Print and shaded views of the part. All mm, measured from the part's lowest x, y and z. Give positions to 0.01 mm unless a question says otherwise; leave off trailing zeros. Write each loop counter-clockwise with the first axis right and the second up, starting at its lowest first coordinate (ties: lowest second). Pieces come first, ordered by that corner, then holes. Notation, with made-up numbers: M 9,21 L 32,21 A29 cw 32,57 Z; hole C 46,15 d1. An arc over 180 degrees is marked long. One line per question, with ' | ' between items. Start each with the question number.
1. Wall check: L1, parallel to Y at x = 31, z = 1.4; L2, parallel to X at y = 12, z = 3.1; L3, parallel to X at y = 14, z = 1.95. Give the ranges that are in metal, low to high.
2. Flat gauge pins, fed straight in: pin 1 (3.5 mm diameter, centred on x = 39.5, y = 17.5, fed in from +Z); pin 2 (8 mm diameter, centred on x = 12.5, y = 25, fed in from +Z). Where does each tip first touch, or does it go through?
3. Cut at D-D, the plane y = 8. Write the cut outline in (x, z).
4. Cut at A-A, the plane z = 0.45. Write the cut outline in (x, y).
5. Cut at C-C, the plane x = 23.5. Write the cut outline in (y, z), then the cut area to 3 significant figures.
6. Cut at B-B, the plane y = 17.5. Write the cut outline in (x, z).
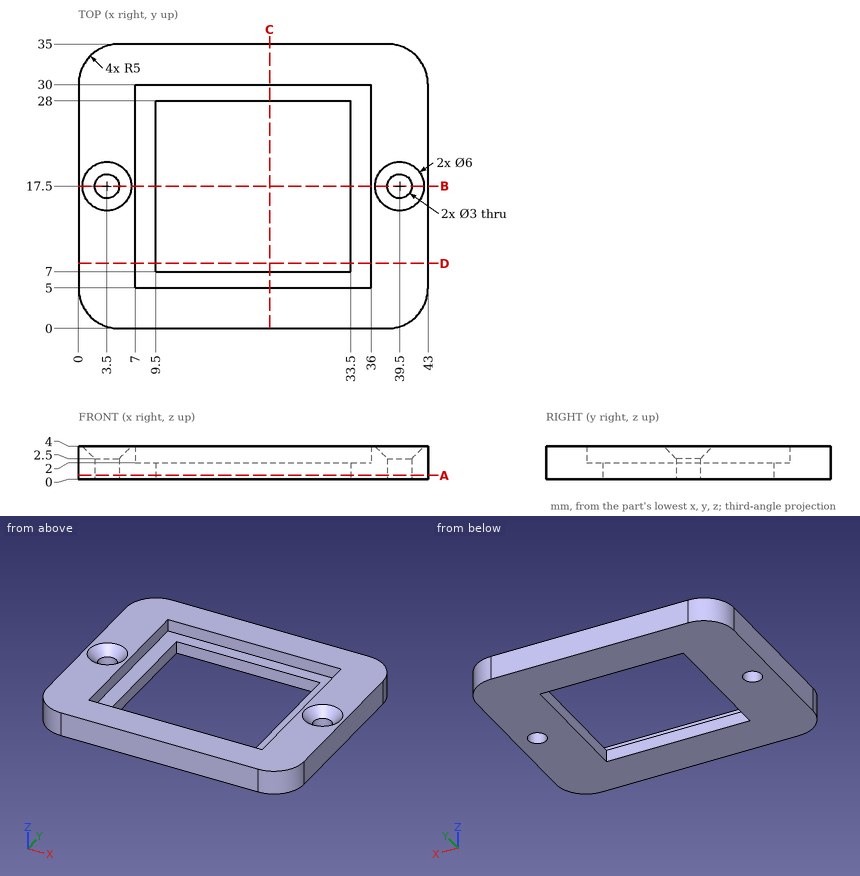
Here are the results:
1) L1: 0 to 7, 28 to 35 | L2: 0 to 7, 36 to 43 | L3: 0 to 9.5, 33.5 to 43
2) pin 1: z = 2.75 | pin 2: z = 2
3) outline: M 0,0 L 9.5,0 L 9.5,2 L 7,2 L 7,4 L 0,4 Z; M 33.5,0 L 43,0 L 43,4 L 36,4 L 36,2 L 33.5,2 Z
4) outline: M 0,5 A5 ccw 5,0 L 38,0 A5 ccw 43,5 L 43,30 A5 ccw 38,35 L 5,35 A5 ccw 0,30 Z; hole C 3.5,17.5 d3; hole M 9.5,7 L 33.5,7 L 33.5,28 L 9.5,28 Z; hole C 39.5,17.5 d3
5) outline: M 0,0 L 7,0 L 7,2 L 5,2 L 5,4 L 0,4 Z; M 28,0 L 35,0 L 35,4 L 30,4 L 30,2 L 28,2 Z | area: 48.0 mm^2
6) outline: M 0,0 L 2,0 L 2,2.5 L 0.5,4 L 0,4 Z; M 5,0 L 9.5,0 L 9.5,2 L 7,2 L 7,4 L 6.5,4 L 5,2.5 Z; M 33.5,0 L 38,0 L 38,2.5 L 36.5,4 L 36,4 L 36,2 L 33.5,2 Z; M 41,0 L 43,0 L 43,4 L 42.5,4 L 41,2.5 Z
